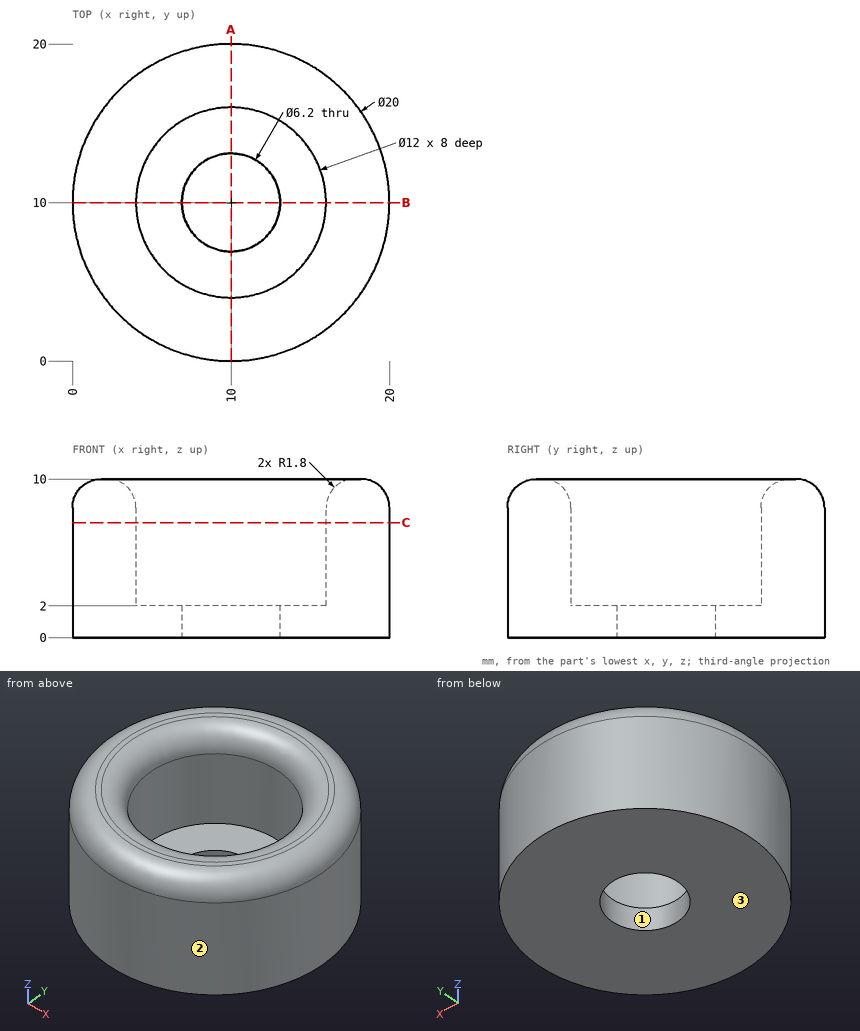
Design review of the part shown in the three views and the two pictorial views. Dimensions are in mm from the part's minimum x, y and z. Coordinates: 2 decimals unless noted, no trailing zeros. Write each loop counter-clockwise with the first axis right and the second up, starting at its lowest first coordinate (ties: lowest second). Pieces come first, ordered by that corner, then holes.
(1) Add section A-A on x = 10. Give the boundary of the cut face in (y, z), then the cut area to 3 significant figures.
(2) For pin 1 Ø5 at (x, y) = (7.5, 6.5) entering from +Z; pin 2 Ø1 at (y, z) = (7.5, 5) entering from -X; pin 3 Ø7 at (x, y) = (10, 10) entering from +Z, all flat-tipped, find the tip position at first contact; note any pin that passes through.
(3) Wall thickness on probe 1 along Y at (x, z) = (10, 1.1); probe 2 along Y at (x, z) = (10, 5.75); probe 3 along Z at (x, y) = (9.75, 14.25): over which ranges is each line inside the solid? List them lowest first.
(4) The part is to be moulded in two halves that separate along X. For the marked faces 1, 2 and 3, say which applies: +X half, -X half, draft (parallel to the pull), parting line (faces both ways), or undercut.
(5) Add section C-C on z = 7.25. Give the boundary of the cut face in (x, y).
Answer sheet:
1. outline: (0, 0) - (6.9, 0) - (6.9, 2) - (4, 2) - (4, 8.2) arc R1.8 ccw to (2.2, 10) - (1.8, 10) arc R1.8 ccw to (0, 8.2) - close; (13.1, 0) - (20, 0) - (20, 8.2) arc R1.8 ccw to (18.2, 10) - (17.8, 10) arc R1.8 ccw to (16, 8.2) - (16, 2) - (13.1, 2) - close
1. area: 88.8 mm2
2. pin 1: stops at z = 9.7
2. pin 2: stops at x = 0.2
2. pin 3: stops at z = 2
3. probe 1: y = 0 to 6.9, 13.1 to 20
3. probe 2: y = 0 to 4, 16 to 20
3. probe 3: z = 0 to 2
4. face 1: undercut
4. face 2: parting line
4. face 3: draft
5. outline: circle Ø20 at (10, 10); hole circle Ø12 at (10, 10)
